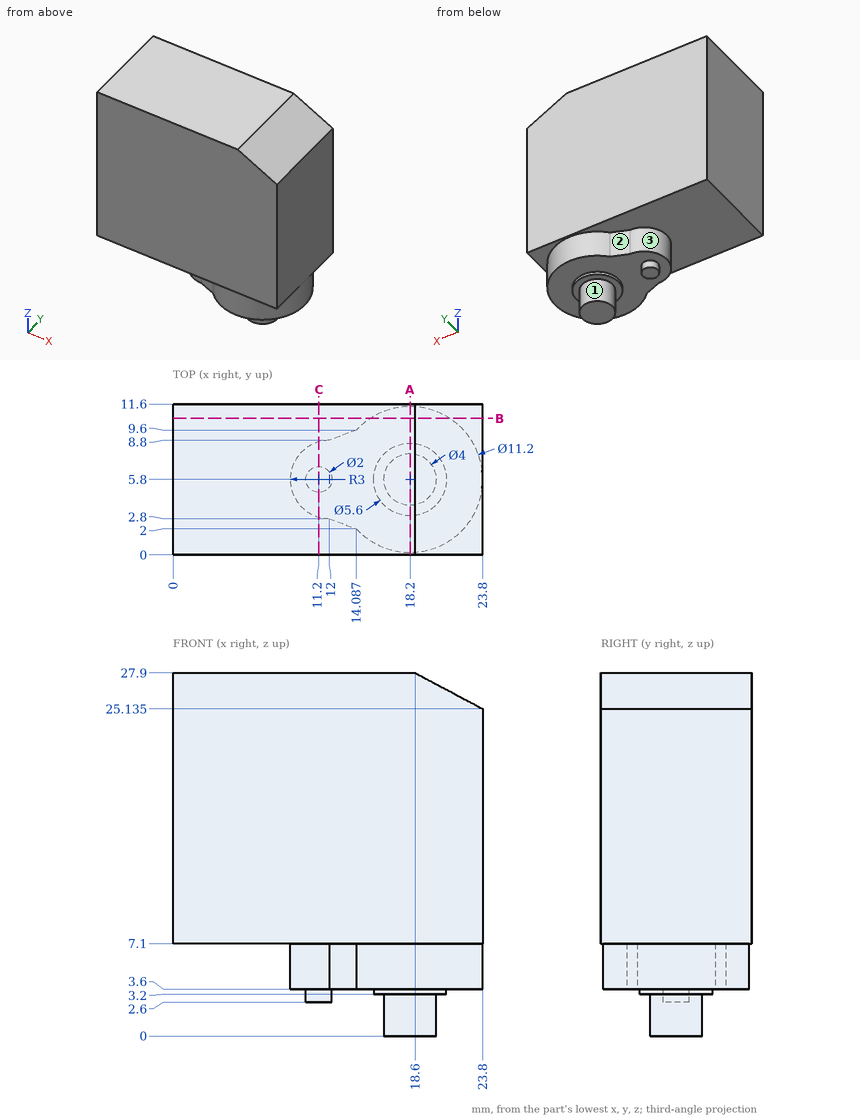
Can you work these out from the drawing? Everything is in mm from the part's minimum corner. A direction names the side the tool comes from. Round coordinates to 2 decimals unless told otherwise and drop trailing zeros. Loops run counter-clockwise (first coordinate to the right, second up) from the corner with the lowest first, then second, coordinate; pieces in that order, holes last. Notation, with made-up numbers: M -40,-13.75 L -20,-13.75 A22 cw -20,25.25 Z; hole C -32.75,55 d9. An arc over 180 degrees is marked long. Answer in a Markdown table with one row per item.
1. If we section it at C-C, the plane x = 11.2: Please give me the cut outline in (y, z).
Established:
| item | result |
|---|---|
| outline | M 0,7.1 L 2.91,7.1 L 2.91,3.6 L 4.8,3.6 L 4.8,2.6 L 6.8,2.6 L 6.8,3.6 L 8.69,3.6 L 8.69,7.1 L 11.6,7.1 L 11.6,27.9 L 0,27.9 Z |
2. If we section it at B-B, the plane y = 10.5: Please give me the cut outline in (x, z) (1 decimal).
Established:
| item | result |
|---|---|
| outline | M 0,7.1 L 15.2,7.1 L 15.2,3.6 L 21.2,3.6 L 21.2,7.1 L 23.8,7.1 L 23.8,25.1 L 18.6,27.9 L 0,27.9 Z |
3. On a 3-axis mill with a long thin cutter (end or side, diameter ignored), from which of +Z, -Z, +X, -X, +Y, -Y can I reach the whole of each face in a straight line? I mean the marked faces 1, 2 and 3. Say none if no direction works.
Established:
| item | result |
|---|---|
| face 1 | -Z |
| face 2 | -Z, -X, +Y |
| face 3 | -Z, -X |
4. Please list where these lines run through material, in increasing order: line 1 (Z direction, x = 2.75, y = 10.25); line 2 (Z direction, x = 9.75, y = 5.25); line 3 (Y direction, x = 15, z = 5.75) (1 decimal). Write a range as from..to.
Established:
| item | result |
|---|---|
| line 1 | 7.1..27.9 |
| line 2 | 3.6..27.9 |
| line 3 | 1.2..10.4 |
5. I'm going to push flat-ended pins straight in: pin 1 Ø1 at (x, y) = (11, 5.5) entering from -Z; pin 2 Ø2 at (x, y) = (10.5, 10) entering from -Z. Where does each tip first touch, or does it pass through?
Established:
| item | result |
|---|---|
| pin 1 | z = 2.6 |
| pin 2 | z = 7.1 |
6. If we section it at A-A, the plane x = 18.2: Please give me the cut outline in (y, z).
Established:
| item | result |
|---|---|
| outline | M 0,7.1 L 0.2,7.1 L 0.2,3.6 L 3,3.6 L 3,3.2 L 3.8,3.2 L 3.8,0 L 7.8,0 L 7.8,3.2 L 8.6,3.2 L 8.6,3.6 L 11.4,3.6 L 11.4,7.1 L 11.6,7.1 L 11.6,27.9 L 0,27.9 Z |
